```python
from build123d import *

# Parameters (mm, degrees)
SKETCH1_R           = 30
BOSS_EXTRUDE1_DEPTH = 75
SKETCH2_R           = 25
BOSS_EXTRUDE2_DEPTH = 30
CUT_EXTRUDE1_DEPTH  = 76
FILLET1_R           = 20


with BuildPart() as part:
    # Sketch1 → Boss-Extrude1 (new body, symmetric)
    with BuildSketch(Plane.XY):
        with BuildLine():
            Line((58.094750193, 15), (225, 15))
            Line((225, 15), (225, -15))
            Line((225, -15), (58.094750193, -15))
            ThreePointArc((58.094750193, -15), (-60, 0), (58.094750193, 15))
        make_face()
        Circle(SKETCH1_R, mode=Mode.SUBTRACT)
    extrude(amount=BOSS_EXTRUDE1_DEPTH, both=True)

    # Sketch2 → Boss-Extrude2 (add)
    with BuildSketch(Plane(origin=(0, 0, -75), x_dir=(-1, 0, 0), z_dir=(0, 0, -1))):
        with BuildLine():
            Line((-225, 15), (-225, 55))
            ThreePointArc((-225, 55), (-187.914926762, 103.30325731), (-131.671813331, 79.953321221))
            ThreePointArc((-131.671813331, 79.953321221), (-86.383524737, 45.01789196), (-29.635348145, 52.170356912))
            ThreePointArc((-29.635348145, 52.170356912), (-47.639808951, 36.475314984), (-58.094750193, 15))
            Line((-58.094750193, 15), (-225, 15))
        make_face()
        with Locations((-175, 55)):
            Circle(SKETCH2_R, mode=Mode.SUBTRACT)
    extrude(amount=-BOSS_EXTRUDE2_DEPTH)

    # Sketch3 → Cut-Extrude1 (cut, through all)
    with BuildSketch(Plane(origin=(0, 15, 0), x_dir=(1, 0, 0), z_dir=(0, 1, 0))):
        Polygon((225, 25), (105.824640741, -75), (225, -75), align=None)
    extrude(amount=-CUT_EXTRUDE1_DEPTH, mode=Mode.SUBTRACT)

    # Fillet1
    fillet1_edges = [part.edges().sort_by_distance(p)[0] for p in [
        (225, 0, -25),
        (105.824640741, 0, 75),
    ]]
    fillet(fillet1_edges, radius=FILLET1_R)


solid = part.part
```
Work out the finished part from the listing and answer in its coordinate system (mm). A direction names the side the tool comes from. Round coordinates to 2 decimals unless told otherwise and drop trailing zeros. Write each loop counter-clockwise with the first axis right and the second up, starting at its lowest first coordinate (ties: lowest second). Pieces come first, ordered by that corner, then holes. Notation, with made-up numbers: (-28.75, -21.5) - (-22.75, -21.5) arc R20 cw to (-22.75, 0.5) - close; hole circle Ø2 at (41.5, -22.75). An arc over 180 degrees is marked (long way). Return JSON: item names as keys, results as strings. Group by question number.
Q1. The part is cut by section D-D on x = 175. Write down the section's boundary in (y, z), then the cut area to 3 significant figures.
Q2. Each of these flat-tipped pins is pushed along its axis until it touches: pin 1 Ø2 at (x, z) = (-10, 2.5) entering from +Y; pin 2 Ø5 at (y, z) = (1, 39.5) entering from +X; pin 3 Ø8 at (y, z) = (-28, 47.5) entering from +X. Where does it stop, or does it pass through?
Q3. The part is cut by section A-A on x = 0. Write down the section's boundary in (y, z).
Q4. The mould has two halves that part along Y. Classify faces 1 (the flat face through (124, -15, -16)), 2 (the cylindrical face through (151.91, 45.42, -60.21)), 3 (the cylindrical face through (-29.97, 1.32, -1.05)), 4 (the flat face through (225, 20, -55)): released by +Y, released by -Y, zero draft, split by the parting line, or undercut.
Q5. The part is cut by section C-C on z = -52.5. Write down the section's boundary in (x, y).
Q6. The part is cut by section B-B on y = 0. Write down the section's boundary in (x, z).
Q7. Find the intervals of material crossed by L1, parallel to Y at x = 0, z = 13; L2, parallel to Y at x = 108, z = 31; L3, parallel to Y at x = 22, z = -50, in increasing order.
Q8. For faces 5 (the flat face through (148, 51, -45)), 6 (the cylindrical face through (223.177, -0.21, -25.985)), determine the directions among +Z, -Z, +X, -X, +Y, -Y from which every point of the face is accessible in a straight line to the end or side of a thin tool.
Solved:
{
 "1": {"outline": "(-15, -75) - (30, -75) - (30, -45) - (15, -45) - (15, 16.95) - (-15, 16.95) - close; (80, -75) - (105, -75) - (105, -45) - (80, -45) - close", "area": "3,960 mm²"},
 "2": {"pin 1": "y = 59.32", "pin 2": "x = 151.11", "pin 3": "x = 54.99"},
 "3": {"outline": "(-60, -75) - (-30, -75) - (-30, 75) - (-60, 75) - close; (30, -75) - (60, -75) - (60, 75) - (30, 75) - close"},
 "4": {"face 1": "released by -Y", "face 2": "undercut", "face 3": "undercut", "face 4": "zero draft"},
 "5": {"outline": "(29.64, 52.17) arc R60 ccw (long way) to (58.09, -15) - (225, -15) - (225, 55) arc R50 ccw to (131.67, 79.95) arc R75 cw to start; hole circle Ø60 at (0, 0); hole circle Ø50 at (175, 55)"},
 "6": {"outline": "(-60, -75) - (-30, -75) - (-30, 75) - (-60, 75) - close; (30, -75) - (225, -75) - (225, -34.33) arc R20 ccw to (217.86, -19.01) - (111.4, 70.32) arc R20 ccw to (98.55, 75) - (30, 75) - close"},
 "7": {"L1": "-60 to -30, 30 to 60", "L2": "-15 to 15", "L3": "-55.82 to -20.4, 20.4 to 55.82"},
 "8": {"face 5": "+Z, +X, +Y", "face 6": "+Z, +X, +Y, -Y"}
}
